Read the model definition and answer for the solid it produces. Units are mm, in the model's axes. A direction names the side the tool comes from. Give positions to 0.01 mm unless a question says otherwise; leave off trailing zeros. Order: outer loops, then holes, each group sorted by start corner. A loop starts at its lowest first (then second) coordinate and runs counter-clockwise, first axis right, second up.
Item 1: Find the intervals of material crossed by line 1 along X through (y, z) = (-2.1, 0.2); line 2 along X through (y, z) = (1.7, 0.3); line 3 along Y through (x, z) = (2.5, 0.45), in increasing order.
Item 2: A cutting plane is placed at A-A (y = 2.3). Write down the section's boundary in (x, z).
Item 3: A cutting plane is placed at C-C (y = -2). Write down the section's boundary in (x, z), plus the area to 3 significant figures.
Item 4: The mould has two halves that part along Y. Classify faces 4 (the face through (-2.003, 1.296, 0.246)), 5 (the face through (-1.283, 1.991, 0.246)), 6 (the face through (0, 0, 0.5)): +Y half, -Y half, draft (parallel to the pull), parting line (faces both ways), or undercut.
Item 5: A cutting plane is placed at B-B (y = 1.15). Write down the section's boundary in (x, z), plus the area to 3 significant figures.
Item 6: Which of the six approach directions +Z, -Z, +X, -X, +Y, -Y give full straight-line access (tool end or side, diameter ignored) to faces 1 (the face through (1.296, 2.003, 0.246)), 2 (the face through (-1.991, -1.283, 0.246)), 3 (the face through (1.283, -1.991, 0.246))?
from build123d import *

# Parameters (mm, degrees)
F1_DEPTH = 0.5


with BuildPart() as f1:
    # F0 (on Top) → F1 (new body)
    with BuildSketch(Plane.XY):
        with BuildLine():
            Line((0.5, 1.689949), (0.5, 2.95804))
            ThreePointArc((0.5, 2.95804), (0, 3), (-0.5, 2.95804))
            Line((-0.5, 2.95804), (-0.5, 1.689949))
            ThreePointArc((-0.5, 1.689949), (-0.623463, 1.505174), (-0.841421, 1.548528))
            Line((-0.841421, 1.548528), (-1.738097, 2.445203))
            ThreePointArc((-1.738097, 2.445203), (-2.12132, 2.12132), (-2.445203, 1.738097))
            Line((-2.445203, 1.738097), (-1.548528, 0.841421))
            ThreePointArc((-1.548528, 0.841421), (-1.505174, 0.623463), (-1.689949, 0.5))
            Line((-1.689949, 0.5), (-3, 0.5))
            Line((-3, 0.5), (-3, 1.25))
            Line((-3, 1.25), (-3.8, 1.25))
            Line((-3.8, 1.25), (-3.8, -1.25))
            Line((-3.8, -1.25), (-3, -1.25))
            Line((-3, -1.25), (-3, -0.5))
            Line((-3, -0.5), (-1.689949, -0.5))
            ThreePointArc((-1.689949, -0.5), (-1.505174, -0.623463), (-1.548528, -0.841421))
            Line((-1.548528, -0.841421), (-2.445203, -1.738097))
            ThreePointArc((-2.445203, -1.738097), (-2.12132, -2.12132), (-1.738097, -2.445203))
            Line((-1.738097, -2.445203), (-0.841421, -1.548528))
            ThreePointArc((-0.841421, -1.548528), (-0.623463, -1.505174), (-0.5, -1.689949))
            Line((-0.5, -1.689949), (-0.5, -2.95804))
            ThreePointArc((-0.5, -2.95804), (0, -3), (0.5, -2.95804))
            Line((0.5, -2.95804), (0.5, -1.689949))
            ThreePointArc((0.5, -1.689949), (0.623463, -1.505174), (0.841421, -1.548528))
            Line((0.841421, -1.548528), (1.738097, -2.445203))
            ThreePointArc((1.738097, -2.445203), (2.12132, -2.12132), (2.445203, -1.738097))
            Line((2.445203, -1.738097), (1.548528, -0.841421))
            ThreePointArc((1.548528, -0.841421), (1.505174, -0.623463), (1.689949, -0.5))
            Line((1.689949, -0.5), (2.95804, -0.5))
            ThreePointArc((2.95804, -0.5), (3, 0), (2.95804, 0.5))
            Line((2.95804, 0.5), (1.689949, 0.5))
            ThreePointArc((1.689949, 0.5), (1.505174, 0.623463), (1.548528, 0.841421))
            Line((1.548528, 0.841421), (2.445203, 1.738097))
            ThreePointArc((2.445203, 1.738097), (2.12132, 2.12132), (1.738097, 2.445203))
            Line((1.738097, 2.445203), (0.841421, 1.548528))
            ThreePointArc((0.841421, 1.548528), (0.623463, 1.505174), (0.5, 1.689949))
        make_face()
    extrude(amount=F1_DEPTH)


solid = f1.part
Response values:
1. line 1: x = -2.14 to -1.39, -0.5 to 0.5, 1.39 to 2.14
1. line 2: x = -2.41 to -0.99, -0.5 to 0.5, 0.99 to 2.41
1. line 3: y = -0.5 to 0.5
2. outline: (-1.93, 0) - (-1.59, 0) - (-1.59, 0.5) - (-1.93, 0.5) - close; (-0.5, 0) - (0.5, 0) - (0.5, 0.5) - (-0.5, 0.5) - close; (1.59, 0) - (1.93, 0) - (1.93, 0.5) - (1.59, 0.5) - close
3. outline: (-2.24, 0) - (-1.29, 0) - (-1.29, 0.5) - (-2.24, 0.5) - close; (-0.5, 0) - (0.5, 0) - (0.5, 0.5) - (-0.5, 0.5) - close; (1.29, 0) - (2.24, 0) - (2.24, 0.5) - (1.29, 0.5) - close
3. area: 1.44 mm2
4. face 4: undercut
4. face 5: +Y half
4. face 6: draft
5. outline: (-3.8, 0) - (-3, 0) - (-3, 0.5) - (-3.8, 0.5) - close; (-1.86, 0) - (1.86, 0) - (1.86, 0.5) - (-1.86, 0.5) - close
5. area: 2.26 mm2
6. face 1: +Z, -Z, +Y
6. face 2: +Z, -Z
6. face 3: +Z, -Z, -Y
